Build history of the part. All positions in model axes, mm. A direction names the side the tool comes from. Round coordinates to 2 decimals unless told otherwise and drop trailing zeros. Write each loop counter-clockwise with the first axis right and the second up, starting at its lowest first coordinate (ties: lowest second). Pieces come first, ordered by that corner, then holes. Notation, with made-up numbers: M 63,77 L 105,77 A9 ccw 105,94 Z; hole C 65,19.5 d9. An arc over 180 degrees is marked long. One line per item, written item: value. Start each with the question number.
```python
from build123d import *

# Parameters (mm, degrees)
F0_R     = 33
F0_R_2   = 0.75
F0_R_3   = 30
F1_DEPTH = 60
F2_DEPTH = 3
F3_T     = -2.5


with BuildPart() as f1:
    # F0 (on Front) → F1 (new body)
    with BuildSketch(Plane.XZ):
        Circle(F0_R)
        with Locations((0, -31.744543)):
            Circle(F0_R_2, mode=Mode.SUBTRACT)
        with Locations((-25.660656, 17.90996)):
            Circle(F0_R_2, mode=Mode.SUBTRACT)
        Circle(F0_R_3, mode=Mode.SUBTRACT)
        with Locations((23.63484, 20.465862)):
            Circle(F0_R_2, mode=Mode.SUBTRACT)
        Circle(F0_R_3)
    extrude(amount=F1_DEPTH)

    # F0 (on Front) → F2 (join)
    with BuildSketch(Plane.XZ):
        Circle(F0_R)
        with Locations((0, -31.744543)):
            Circle(F0_R_2, mode=Mode.SUBTRACT)
        with Locations((-25.660656, 17.90996)):
            Circle(F0_R_2, mode=Mode.SUBTRACT)
        Circle(F0_R_3, mode=Mode.SUBTRACT)
        with Locations((23.63484, 20.465862)):
            Circle(F0_R_2, mode=Mode.SUBTRACT)
    extrude(amount=F2_DEPTH)

    # F3
    f3_openings = [f1.faces().sort_by_distance(p)[0] for p in [
        (0.001048, 0, -0.003431),
    ]]
    offset(amount=F3_T, openings=f3_openings)


solid = f1.part
```
Item 1: Drop flat-ended pins along their axis: pin 1 (3 mm diameter, centred on x = 23.5, y = -42.5, fed in from +Z); pin 2 (0.9 mm diameter, centred on x = -25.66, z = 17.91, fed in from +Y); pin 3 (4 mm diameter, centred on x = 16, z = 4.5, fed in from +Y); pin 4 (5 mm diameter, centred on y = -54, z = 26, fed in from -X). Give the stop position or say it passes through.
Item 2: Cut at B-B, the plane x = -8. Write the cut outline in (y, z).
Item 3: Cut at C-C, the plane y = -47. Write the cut outline in (x, z).
Item 4: Which spindle directions (+Z, -Z, +X, -X, +Y, -Y) get a long thin tool onto all of the face, cutting with end or side? Do faces 1 (the cylindrical face through (-1.25, -28.348, 30.474)), 2 (the flat face through (22, 0, 20)). Say none if no direction does.
Item 5: Drill centre lines: line 1 (Z direction, x = 0, y = -40); line 2 (X direction, y = -19, z = 0.5); line 3 (Y direction, x = 3, z = -8.5). Where is each one in solid material? Low to high.
Item 6: Cut at A-A, the plane z = 0. Write the cut outline in (x, y).
Item 7: Two-plate mould, pull along X, no slides. Class faces 3 (the cylindrical face through (-23.03, -28.35, 16)), 4 (the flat face through (0, -60, 0)), 5 (the cylindrical face through (30.5, -29.6, -12.6)): pulls with the +X half, pulls with the -X half, needs draft (parallel to the pull), parting line crosses it, or undercut.
Computed values:
1. pin 1: stops at z = 24.6
1. pin 2: passes through
1. pin 3: stops at y = -57.5
1. pin 4: stops at x = -23.17
2. outline: M -60,-32.02 L 0,-32.02 L 0,-29.43 L -57.5,-29.43 L -57.5,29.43 L 0,29.43 L 0,32.02 L -60,32.02 Z
3. outline: C 0,0 d66; hole M -26.66,14.82 A30.5 ccw -2.94,-30.36 A3.25 cw 2.94,-30.36 A30.5 ccw 24.98,17.51 A3.25 cw 20.9,22.22 A30.5 ccw -23.1,19.91 A3.25 cw Z; hole C -25.66,17.91 d1.5; hole C 0,-31.74 d1.5; hole C 23.63,20.47 d1.5
4. face 1: +Y
4. face 2: +Z, -Z, +X, -X, +Y
5. line 1: z = -33 to -32.49, -30.99 to -28.49, 30.5 to 33
5. line 2: x = -33 to -30.5, 30.5 to 33
5. line 3: y = -60 to -57.5
6. outline: M -33,-60 L 33,-60 L 33,0 L 30.5,0 L 30.5,-57.5 L -30.5,-57.5 L -30.5,0 L -33,0 Z
7. face 3: undercut
7. face 4: needs draft
7. face 5: parting line crosses it
